```python
from build123d import *

# Parameters (mm, degrees)
SKETCH_1_W          = 20
SKETCH_1_H          = 48
EXTRUDE_2_DEPTH     = 4
SKETCH_3_W          = 20
SKETCH_3_H          = 3
EXTRUDE_3_DEPTH     = 8
SKETCH_4_W          = 12
SKETCH_4_H          = 4
EXTRUDE_4_DEPTH     = 15
SKETCH_5_R          = 1.75
CUT_EXTRUDE_2_DEPTH = 37.674241642
SKETCH_6_W          = 12
SKETCH_6_H          = 12
SKETCH_6_R          = 1.75
EXTRUDE_5_DEPTH     = 20
SKETCH_7_W          = 10
SKETCH_7_H          = 48
EXTRUDE_6_DEPTH     = 20
SKETCH_8_R          = 1.65
CUT_EXTRUDE_3_DEPTH = 46.299006612
CHAMFER_1_SIZE      = 3
FILLET_2_R          = 2.5
SKETCH_11_W         = 8
SKETCH_11_H         = 12
CUT_EXTRUDE_5_DEPTH = 3
SKETCH_12_R         = 1.4
CUT_EXTRUDE_6_DEPTH = 60.203040462
CHAMFER_2_SIZE      = 1.5
SKETCH_14_W         = 21.274376693
SKETCH_14_H         = 42.4
CUT_EXTRUDE_7_DEPTH = 8
SKETCH_15_W         = 103.642401021
SKETCH_15_H         = 66.860791826
CUT_EXTRUDE_8_DEPTH = 106


with BuildPart() as part:
    # 草图1 → 凸台-拉伸2 (new body)
    with BuildSketch(Plane(origin=(0, 0, 0), x_dir=(1, 0, 0), z_dir=(0, 1, 0))):
        Rectangle(SKETCH_1_W, SKETCH_1_H)
    extrude(amount=EXTRUDE_2_DEPTH)

    # 草图3 → 凸台-拉伸3 (add)
    with BuildSketch(Plane.XZ):
        with Locations((0, 22.5)):
            Rectangle(SKETCH_3_W, SKETCH_3_H)
        with Locations((0, -22.5)):
            Rectangle(SKETCH_3_W, SKETCH_3_H)
    extrude(amount=EXTRUDE_3_DEPTH)

    # 草图4 → 凸台-拉伸4 (add)
    with BuildSketch(Plane.ZY.offset(10)):
        with Locations((-15, 2)):
            Rectangle(SKETCH_4_W, SKETCH_4_H)
    extrude(amount=EXTRUDE_4_DEPTH)

    # 草图5 → 切除-拉伸2 (cut, through all)
    with BuildSketch(Plane(origin=(0, 4, 0), x_dir=(1, 0, 0), z_dir=(0, 1, 0))):
        with Locations(Location((-19.1, 13, 0), (0, 0, 270))):
            Circle(SKETCH_5_R)
    extrude(amount=-CUT_EXTRUDE_2_DEPTH, mode=Mode.SUBTRACT)

    # 草图6 → 凸台-拉伸5 (add)
    with BuildSketch(Plane.XZ):
        with Locations((-19, -15)):
            Rectangle(SKETCH_6_W, SKETCH_6_H)
        with Locations(Location((-19.1, -13, 0), (0, 0, 90))):
            Circle(SKETCH_6_R, mode=Mode.SUBTRACT)
    extrude(amount=EXTRUDE_5_DEPTH)

    # 草图7 → 凸台-拉伸6 (add)
    with BuildSketch(Plane(origin=(0, 4, 0), x_dir=(1, 0, 0), z_dir=(0, 1, 0))):
        Rectangle(SKETCH_7_W, SKETCH_7_H)
    extrude(amount=EXTRUDE_6_DEPTH)

    # 草图8 → 切除-拉伸3 (cut, through all)
    with BuildSketch(Plane(origin=(5, 0, 0), x_dir=(0, 0, -1), z_dir=(1, 0, 0))):
        with Locations((-18, 19)):
            Circle(SKETCH_8_R)
        with Locations((18, 19)):
            Circle(SKETCH_8_R)
        with Locations((18, 9)):
            Circle(SKETCH_8_R)
        with Locations((-18, 9)):
            Circle(SKETCH_8_R)
    extrude(amount=-CUT_EXTRUDE_3_DEPTH, mode=Mode.SUBTRACT)

    # 倒角1
    chamfer_1_edges = [part.edges().sort_by_distance(p)[0] for p in [
        (-10, -2, -24),
    ]]
    chamfer(chamfer_1_edges, length=CHAMFER_1_SIZE - 0.0001)  # a hair under: the kernel refuses the full size

    # 圆角2
    fillet_2_edges = [part.edges().sort_by_distance(p)[0] for p in [
        (-13, 0, -15),
    ]]
    fillet(fillet_2_edges, radius=FILLET_2_R)

    # 草图11 → 切除-拉伸5 (cut)
    with BuildSketch(Plane(origin=(0, 0, -24), x_dir=(-1, 0, 0), z_dir=(0, 0, -1))):
        with Locations((6, -2)):
            Rectangle(SKETCH_11_W, SKETCH_11_H)
    extrude(amount=-CUT_EXTRUDE_5_DEPTH, mode=Mode.SUBTRACT)

    # 草图12 → 切除-拉伸6 (cut, through all)
    with BuildSketch(Plane.XY.offset(24)):
        with Locations((2, -4.5)):
            Circle(SKETCH_12_R)
    extrude(amount=-CUT_EXTRUDE_6_DEPTH, mode=Mode.SUBTRACT)

    # 倒角2
    chamfer_2_edges = [part.edges().sort_by_distance(p)[0] for p in [
        (0.6, -4.5, 24),
    ]]
    chamfer(chamfer_2_edges, length=CHAMFER_2_SIZE)

    # 草图14 → 切除-拉伸7 (cut)
    with BuildSketch(Plane.XZ.offset(8)):
        with Locations((0.637188347, 0)):
            Rectangle(SKETCH_14_W, SKETCH_14_H)
    extrude(amount=-CUT_EXTRUDE_7_DEPTH, mode=Mode.SUBTRACT)


with BuildPart() as body_2:
    # 镜向2: mirrored copy
    add(part.part.mirror(Plane(origin=(0, 0, -34), x_dir=(1, 0, 0), z_dir=(0, 0, -1))))


with BuildPart() as part_1:
    add(part.part)

    # 草图15 → 切除-拉伸8 (cut, through all)
    with BuildSketch(Plane(origin=(0, 24, 0), x_dir=(1, 0, 0), z_dir=(0, 1, 0))):
        with Locations((-18.895114943, 2.939974457)):
            Rectangle(SKETCH_15_W, SKETCH_15_H)
    extrude(amount=-CUT_EXTRUDE_8_DEPTH, mode=Mode.SUBTRACT)


solid = body_2.part
```
Here's how the part is built. I have some questions about the finished solid (model axes, mm). A direction names the side the tool comes from. Coordinates: 2 decimals unless noted, no trailing zeros. Order: outer loops, then holes, each group sorted by start corner. A loop starts at its lowest first (then second) coordinate and runs counter-clockwise, first axis right, second up. Notation, with made-up numbers: M 83.25,88 L 115.25,88 A7 cw 115.25,97 Z; hole C -17.5,36 d5. An arc over 180 degrees is marked long. Answer as a JSON object with one key per item and string values. Group by question number.
(1) Suppose I cut it at C-C, the plane y = 9. Please give me the cut outline in (x, z), then the cut area to 3 significant figures.
(2) Which directions (+Z, -Z, +X, -X, +Y, -Y) give clear straight access to the entire face, cutting with the end or side of a thin tool? Please do faces 4 (the face through (8, 4, -68)), 5 (the face through (0, 0, -68)), 6 (the face through (-2, -2, -45)).
(3) I need wall thicknesses on probe 1 along Y at (x, z) = (2, -45); probe 2 along X at (y, z) = (-9, -55); probe 3 along Y at (x, z) = (-0.75, -86). Which ranges of each line are inside material? Lowest first, please.
(4) Suppose I cut it at A-A, the plane x = 2. Please give me the cut outline in (y, z).
(5) Suppose I cut it at D-D, the plane x = -4. Please give me the cut outline in (y, z).
(6) For pin 1 (1.4 mm diameter, centred on x = 3.5, z = -91, fed in from -Y); pin 2 (6 mm diameter, centred on x = -11, z = -65.5, fed in from +Y); pin 3 (2.5 mm diameter, centred on y = 0.5, z = -45.5, fed in from -X); pin 4 (5 mm diameter, centred on y = 5.5, z = -54.5, fed in from -X), each with a flat end and sliding along its axis, tell me the tip position at first contact or that it passes through.
(7) Suppose I cut it at B-B, the plane y = -4.5. Please give me the cut outline in (x, z).
(8) If we mould it in two halves opening along Z, with no side actions, what happens to faces 1 (the face through (0.07, 20.115, -87.216)), 2 (the face through (-19, -8, -59)), 3 (the face through (0, 24, -68))? For each: released by +Z, released by -Z, zero draft, split by the parting line, or undercut.
Values found:
{
 "1": {"outline": "M -5,-92 L 5,-92 L 5,-87.65 L -5,-87.65 Z; M -5,-84.35 L 5,-84.35 L 5,-51.65 L -5,-51.65 Z; M -5,-48.35 L 5,-48.35 L 5,-44 L -5,-44 Z", "area": "414 mm^2"},
 "2": {"face 4": "+Z, -Z, +X, +Y", "face 5": "+X, -Y", "face 6": "+Z, -X, -Y"},
 "3": {"probe 1": "y = -8 to -5.9, -3.1 to 24", "probe 2": "x = -25 to -20.85, -17.35 to -13", "probe 3": "y = 0 to 7.35, 10.65 to 17.35, 20.65 to 24"},
 "4": {"outline": "M -8,-92 L -7.4,-92 L -5.9,-90.5 L -5.9,-89.2 L -8,-89.2 Z; M -8,-46.8 L -5.9,-46.8 L -5.9,-44 L -8,-44 Z; M -3.1,-90.5 L -1.6,-92 L 24,-92 L 24,-44 L -3.1,-44 L -3.1,-46.8 L 0,-46.8 L 0,-89.2 L -3.1,-89.2 Z; hole C 9,-86 d3.3; hole C 9,-50 d3.3; hole C 19,-86 d3.3; hole C 19,-50 d3.3"},
 "5": {"outline": "M -8,-92 L 24,-92 L 24,-44 L 4,-44 L 4,-47 L 0,-47 L 0,-89.2 L -8,-89.2 Z; hole C 9,-86 d3.3; hole C 9,-50 d3.3; hole C 19,-86 d3.3; hole C 19,-50 d3.3"},
 "6": {"pin 1": "stops at y = -8", "pin 2": "stops at y = 4", "pin 3": "stops at x = -2", "pin 4": "stops at x = -25"},
 "7": {"outline": "M -25,-59 L -13,-59 L -13,-47 L -25,-47 Z; M -10,-92 L -0.9,-92 L 0.6,-90.5 L 0.6,-89.2 L -10,-89.2 Z; M -2,-46.8 L 0.6,-46.8 L 0.6,-44 L -2,-44 Z; M 3.4,-90.5 L 4.9,-92 L 10,-92 L 10,-89.2 L 3.4,-89.2 Z; M 3.4,-46.8 L 10,-46.8 L 10,-44 L 3.4,-44 Z; hole C -19.1,-55 d3.5"},
 "8": {"face 1": "undercut", "face 2": "released by -Z", "face 3": "zero draft"}
}
